For this review, take the finished solid that the model builds, in its own axes (mm). Round coordinates to 2 decimals unless told otherwise and drop trailing zeros. Write each loop counter-clockwise with the first axis right and the second up, starting at its lowest first coordinate (ties: lowest second). Pieces come first, ordered by that corner, then holes. Notation, with made-up numbers: (-26, 48) -> (-17, 48) arc R15 ccw to (-17, 75) -> close; hole circle Ø5 at (80.25, 10). An arc over 180 degrees is marked (long way). Write each question's results on one line, items separated by ' | '. Start each with the question number.
Item 1: Add section C-C (y = 3.25). State the section outline as (x, z) points, plus the area to 3 significant figures.
Item 2: Clearance check with flat-ended pins moving along their axes: pin 1 (4 mm diameter, centred on x = 0, z = -22.5, fed in from +Y); pin 2 (5 mm diameter, centred on y = 1.5, z = -4.5, fed in from +X); pin 3 (3 mm diameter, centred on x = 2, y = 5.5, fed in from +Z). State where each tip first meets the part, or that it passes through.
Item 3: Add section B-B (z = 22.5). State the section outline as (x, y) points, plus the area to 3 significant figures.
Item 4: To check wall thickness, follow line 1 along X through (y, z) = (1.65, -22.5); line 2 along Y through (x, z) = (3.4, -30.5); line 3 along Z through (x, y) = (3.5, 7.75). State the ranges of each line that lie inside material, in increasing order.
Item 5: Add section D-D (y = 6). State the section outline as (x, z) points, plus the area to 3 significant figures.
Item 6: Add section A-A (x = 3.5). State the section outline as (y, z) points, plus the area to 3 significant figures.
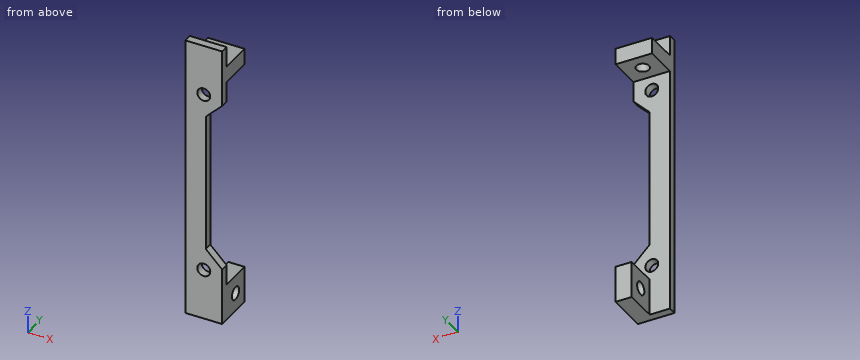
from build123d import *

# Parameters (mm, degrees)
ESBO_O6_W                = 9
ESBO_O6_H                = 70
RESSALTO_EXTRUS_O5_DEPTH = 2
ESBO_O7_W                = 9
ESBO_O7_H                = 4
ESBO_O7_W_2              = 4
ESBO_O7_H_2              = 9
RESSALTO_EXTRUS_O6_DEPTH = 8
ESBO_O8_R                = 1.6
CORTE_EXTRUS_O4_DEPTH    = 5
ESBO_O9_R                = 1.6
CORTE_EXTRUS_O5_DEPTH    = 5
CORTE_EXTRUS_O8_DEPTH    = 37.183559803
ESBO_O12_R               = 1.6
CORTE_EXTRUS_O9_DEPTH    = 5


with BuildPart() as part:
    # Esboço6 → Ressalto-extrusão5 (new body)
    with BuildSketch(Plane(origin=(0, 0, 0), x_dir=(1, 0, 0), z_dir=(0, 1, 0))):
        Rectangle(ESBO_O6_W, ESBO_O6_H)
    extrude(amount=RESSALTO_EXTRUS_O5_DEPTH)

    # Esboço7 → Ressalto-extrusão6 (add)
    with BuildSketch(Plane(origin=(0, 2, 0), x_dir=(1, 0, 0), z_dir=(0, 1, 0))):
        with Locations((0, -28)):
            Rectangle(ESBO_O7_W, ESBO_O7_H)
        with Locations((2.5, 30.5)):
            Rectangle(ESBO_O7_W_2, ESBO_O7_H_2)
    extrude(amount=RESSALTO_EXTRUS_O6_DEPTH)

    # Esboço8 → Corte-extrusão4 (cut)
    with BuildSketch(Plane.XY.offset(30)):
        with Locations((0, 6)):
            Circle(ESBO_O8_R)
    extrude(amount=-CORTE_EXTRUS_O4_DEPTH, mode=Mode.SUBTRACT)

    # Esboço9 → Corte-extrusão5 (cut)
    with BuildSketch(Plane(origin=(4.5, 0, 0), x_dir=(0, 0, -1), z_dir=(1, 0, 0))):
        with Locations((30.5, 6)):
            Circle(ESBO_O9_R)
    extrude(amount=-CORTE_EXTRUS_O5_DEPTH, mode=Mode.SUBTRACT)

    # Esboço10 → Corte-extrusão8 (cut, through all)
    with BuildSketch(Plane(origin=(0, 2, 0), x_dir=(1, 0, 0), z_dir=(0, 1, 0))):
        Polygon((4.5, 21), (0.5, 17), (0.5, -17), (4.5, -21), align=None)
    extrude(amount=-CORTE_EXTRUS_O8_DEPTH, mode=Mode.SUBTRACT)

    # Esboço12 → Corte-extrusão9 (cut)
    with BuildSketch(Plane(origin=(0, 2, 0), x_dir=(1, 0, 0), z_dir=(0, 1, 0))):
        with Locations(Location((0, 22.5, 0), (0, 0, 270))):
            Circle(ESBO_O12_R)
        with Locations(Location((0, -22.5, 0), (0, 0, 270))):
            Circle(ESBO_O12_R)
    extrude(amount=-CORTE_EXTRUS_O9_DEPTH, mode=Mode.SUBTRACT)


solid = part.part
Responses:
1) outline: (-4.5, 26) -> (4.5, 26) -> (4.5, 30) -> (-4.5, 30) -> close; (0.5, -35) -> (4.5, -35) -> (4.5, -26) -> (0.5, -26) -> close | area: 72.0 mm^2
2) pin 1: stops at y = 2 | pin 2: stops at x = 0.5 | pin 3: stops at z = 30
3) outline: (-4.5, 0) -> (-1.6, 0) -> (-1.6, 2) -> (-4.5, 2) -> close; (1.6, 0) -> (4.5, 0) -> (4.5, 2) -> (1.6, 2) -> close | area: 11.6 mm^2
4) line 1: x = -4.5 to -1.6, 1.6 to 4.5 | line 2: y = 0 to 4.4, 7.6 to 10 | line 3: z = -35 to -26, 26 to 30
5) outline: (-4.5, 26) -> (-1.6, 26) -> (-1.6, 30) -> (-4.5, 30) -> close; (0.5, -35) -> (4.5, -35) -> (4.5, -32.1) -> (0.5, -32.1) -> close; (0.5, -28.9) -> (4.5, -28.9) -> (4.5, -26) -> (0.5, -26) -> close; (1.6, 26) -> (4.5, 26) -> (4.5, 30) -> (1.6, 30) -> close | area: 46.4 mm^2
6) outline: (0, -35) -> (10, -35) -> (10, -26) -> (2, -26) -> (2, -20) -> (0, -20) -> close; (0, 20) -> (2, 20) -> (2, 26) -> (10, 26) -> (10, 30) -> (2, 30) -> (2, 35) -> (0, 35) -> close; hole circle Ø3.2 at (6, -30.5) | area: 156 mm^2
